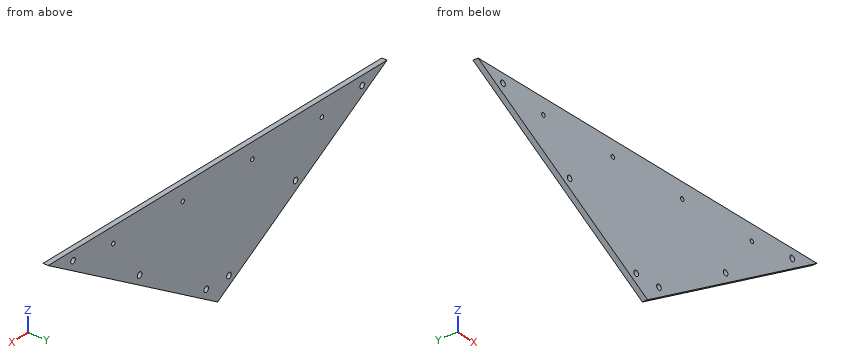
from build123d import *

# Parameters (mm, degrees)
BOSS_EXTRUDE1_DEPTH = 6.35
SKETCH2_R           = 2.4638
CUT_EXTRUDE1_DEPTH  = 7.35
LPATTERN1_COUNT     = 4
LPATTERN1_PITCH     = 101.6
SKETCH3_R           = 3.3655
CUT_EXTRUDE2_DEPTH  = 7.35


with BuildPart() as part:
    # Sketch1 → Boss-Extrude1 (new body)
    with BuildSketch(Plane(origin=(0, 0, 0), x_dir=(1, 0, 0), z_dir=(0, 1, 0))):
        Polygon((0, 0), (247.65, 152.4), (495.3, 0), align=None)
    extrude(amount=BOSS_EXTRUDE1_DEPTH)

    # Sketch2 → Cut-Extrude1 (cut, through all)
    with BuildSketch(Plane(origin=(0, 6.35, 0), x_dir=(1, 0, 0), z_dir=(0, 1, 0))):
        with Locations((95.25, 19.05)):
            Circle(SKETCH2_R)
    cut_extrude1 = extrude(amount=-CUT_EXTRUDE1_DEPTH, mode=Mode.SUBTRACT)

    # LPattern1: Cut-Extrude1 ×4
    with Locations(*[(i * LPATTERN1_PITCH, 0, 0) for i in range(1, LPATTERN1_COUNT)]):
        add(cut_extrude1, mode=Mode.SUBTRACT)

    # Sketch3 → Cut-Extrude2 (cut, through all)
    with BuildSketch(Plane(origin=(0, 6.35, 0), x_dir=(1, 0, 0), z_dir=(0, 1, 0))):
        with Locations((231.009906735, 130.975879922)):
            Circle(SKETCH3_R)
        with Locations((133.665361136, 71.071544168)):
            Circle(SKETCH3_R)
        with Locations((36.320815536, 11.167208415)):
            Circle(SKETCH3_R)
        with Locations((264.290093265, 130.975879922)):
            Circle(SKETCH3_R)
        with Locations((361.634638864, 71.071544168)):
            Circle(SKETCH3_R)
        with Locations((458.979184464, 11.167208415)):
            Circle(SKETCH3_R)
    extrude(amount=-CUT_EXTRUDE2_DEPTH, mode=Mode.SUBTRACT)


solid = part.part
Geometry check sheet. Reference: the model listing, model coordinates, mm. Give positions to 0.01 mm unless a question says otherwise; leave off trailing zeros. Loops run counter-clockwise (first coordinate to the right, second up) from the corner with the lowest first, then second, coordinate; pieces in that order, holes last. Notation, with made-up numbers: M 77.5,72.5 L 90.5,72.5 A28 cw 90.5,94.5 Z; hole C -19,-33.5 d11. An arc over 180 degrees is marked long. Answer as a JSON object with one key per item and string values. Group by question number.
Item 1: Material ranges on L1, parallel to X at y = 3.75, z = -19.05; L2, parallel to X at y = 6, z = -69 (3 decimals); L3, parallel to Z at x = 297.5, y = 1.5, recorded low to high.
Item 2: Gauge pin test, flat ends, axial feed: pin 1 (3 mm diameter, centred on y = 1.5, z = -45.5, fed in from +X); pin 2 (2 mm diameter, centred on y = 1, z = -89.5, fed in from -X). Record the tip position at first contact, or that the pin passes through.
Item 3: Sectioned sample at A-A on y = 3.25. Give the number of separate pieces and of enclosed holes in the cut face, plus the area to 3 significant figures.
Item 4: Sectioned sample at C-C on x = 277. Record the boundary of the cut face in (y, z).
Item 5: Sectioned sample at B-B on z = -88. Record the boundary of the cut face in (x, y), plus the area to 3 significant figures.
Findings below:
{
 "1": {"L1": "30.96 to 92.79, 97.71 to 194.39, 199.31 to 295.99, 300.91 to 397.59, 402.51 to 464.34", "L2": "112.125 to 131.013, 136.318 to 358.982, 364.287 to 383.175", "L3": "-121.72 to -21.32, -16.78 to 0"},
 "2": {"pin 1": "x = 423.8", "pin 2": "x = 143.81"},
 "3": {"separate pieces": "1", "enclosed holes": "10", "area": "37,500 mm2"},
 "4": {"outline": "M 0,-134.34 L 6.35,-134.34 L 6.35,0 L 0,0 Z"},
 "5": {"outline": "M 143,0 L 352.3,0 L 352.3,6.35 L 143,6.35 Z", "area": "1,330 mm2"}
}
